Can you work these out from the model? Positions are in its coordinate system, mm. A direction names the side the tool comes from. Give positions to 0.01 mm unless a question says otherwise; leave off trailing zeros. Write each loop counter-clockwise with the first axis right and the second up, starting at its lowest first coordinate (ties: lowest second). Pieces come first, ordered by that corner, then holes. Notation, with made-up numbers: (5, 58) -> (49, 58) arc R28 ccw to (49, 94) -> close; hole circle Ø11 at (42.25, 2.25). An arc over 180 degrees is marked (long way). One line per item, written item: value.
from build123d import *

# Parameters (mm, degrees)
CROQUIS1_R              = 10
SALIENTE_EXTRUIR1_DEPTH = 6
CROQUIS2_R              = 21
CROQUIS2_R_2            = 10
CORTAR_EXTRUIR1_DEPTH   = 3
CORTAR_EXTRUIR2_DEPTH   = 26
REDONDEO1_R             = 0.5


with BuildPart() as part:
    # Croquis1 → Saliente-Extruir1 (new body)
    with BuildSketch(Plane.XY):
        with BuildLine():
            Line((-5, 20.396078054), (-5, 53))
            Line((-5, 53), (1.774122543, 52.047959163))
            ThreePointArc((1.774122543, 52.047959163), (4.166539486, 50.789247719), (5.211948278, 48.296230713))
            Line((5.211948278, 48.296230713), (6.7, 19.902512404))
            ThreePointArc((6.7, 19.902512404), (-0.88509986, -20.981339286), (-5, 20.396078054))
        make_face()
        Circle(CROQUIS1_R, mode=Mode.SUBTRACT)
    extrude(amount=SALIENTE_EXTRUIR1_DEPTH)

    # Croquis2 → Cortar-Extruir1 (cut)
    with BuildSketch(Plane(origin=(0, 0, 0), x_dir=(-1, 0, 0), z_dir=(0, 0, -1))):
        Circle(CROQUIS2_R)
        Circle(CROQUIS2_R_2, mode=Mode.SUBTRACT)
    extrude(amount=-CORTAR_EXTRUIR1_DEPTH, mode=Mode.SUBTRACT)

    # Croquis3 → Cortar-Extruir2 (cut)
    with BuildSketch(Plane(origin=(0, 53, 0), x_dir=(-1, 0, 0), z_dir=(0, 1, 0))):
        Polygon((5, 6), (5, 1.8), (0, 6), align=None)
    extrude(amount=-CORTAR_EXTRUIR2_DEPTH, mode=Mode.SUBTRACT)

    # Redondeo1
    redondeo1_edges = [part.edges().sort_by_distance(p)[0] for p in [
        (-2.5, 27, 3.9),
    ]]
    fillet(redondeo1_edges, radius=REDONDEO1_R)


solid = part.part
1) For faces 4 (the face through (0, 16, 6)), 5 (the face through (-3, 27, 5)), 6 (the face through (-5, 32.8, 1.6)), which set-ups out of +Z, -Z, +X, -X, +Y, -Y let a thin tool reach every point of the face, with its end or its side?
Answer list:
face 4: +Z, +X, -X, +Y, -Y
face 5: +Z, -X, +Y
face 6: +Z, -Z, -X, +Y
2) I need wall thicknesses on L1, parallel to Y at x = 0, z = 4.35; L2, parallel to Z at x = -9.5, y = -12.5; L3, parallel to X at y = 48.5, z = 0.9. Which ranges of each line are inside material? Lowest first, please.
Answer list:
L1: y = -21 to -10, 10 to 52.3
L2: z = 3 to 6
L3: x = -5 to 5.2
3) If we section it at C-C (y = 47): Write out the boundary of the cut face in (x, z), and give its area (3 significant figures).
Answer list:
outline: (-5, 0) -> (5.28, 0) -> (5.28, 6) -> (0, 6) -> (-5, 1.8) -> close
area: 51.2 mm^2
4) We'd pull the mould along X, two halves only. Please class faces 1 (the face through (0.802, 20.985, 1.479)), 2 (the face through (4.14, 50.82, 2.96)), 3 (the face through (-2.5, 40.4, 3.9)): released by +X, released by -X, zero draft, split by the parting line, or undercut.
Answer list:
face 1: undercut
face 2: released by +X
face 3: released by -X
5) If we section it at A-A (y = 0): Write out the boundary of the cut face in (x, z).
Answer list:
outline: (-21, 3) -> (-10, 3) -> (-10, 6) -> (-21, 6) -> close; (10, 3) -> (21, 3) -> (21, 6) -> (10, 6) -> close
6) If we section it at D-D (x = -13): Write out the boundary of the cut face in (y, z), and give its area (3 significant figures).
Answer list:
outline: (-16.49, 3) -> (16.49, 3) -> (16.49, 6) -> (-16.49, 6) -> close
area: 99.0 mm^2
7) If we section it at B-B (z = 1): Write out the boundary of the cut face in (x, y).
Answer list:
outline: (-5, 20.4) arc R21 cw to (6.7, 19.9) -> (5.21, 48.3) arc R4 ccw to (1.77, 52.05) -> (-5, 53) -> close
8) Will these pins go through, and if not, where does the flat tip stop? pin 1 (1.5 mm diameter, centred on y = 4, z = 5.5, fed in from -X); pin 2 (6 mm diameter, centred on x = -11.5, y = 18.5, fed in from -Z).
Answer list:
pin 1: stops at x = -20.75
pin 2: stops at z = 3
